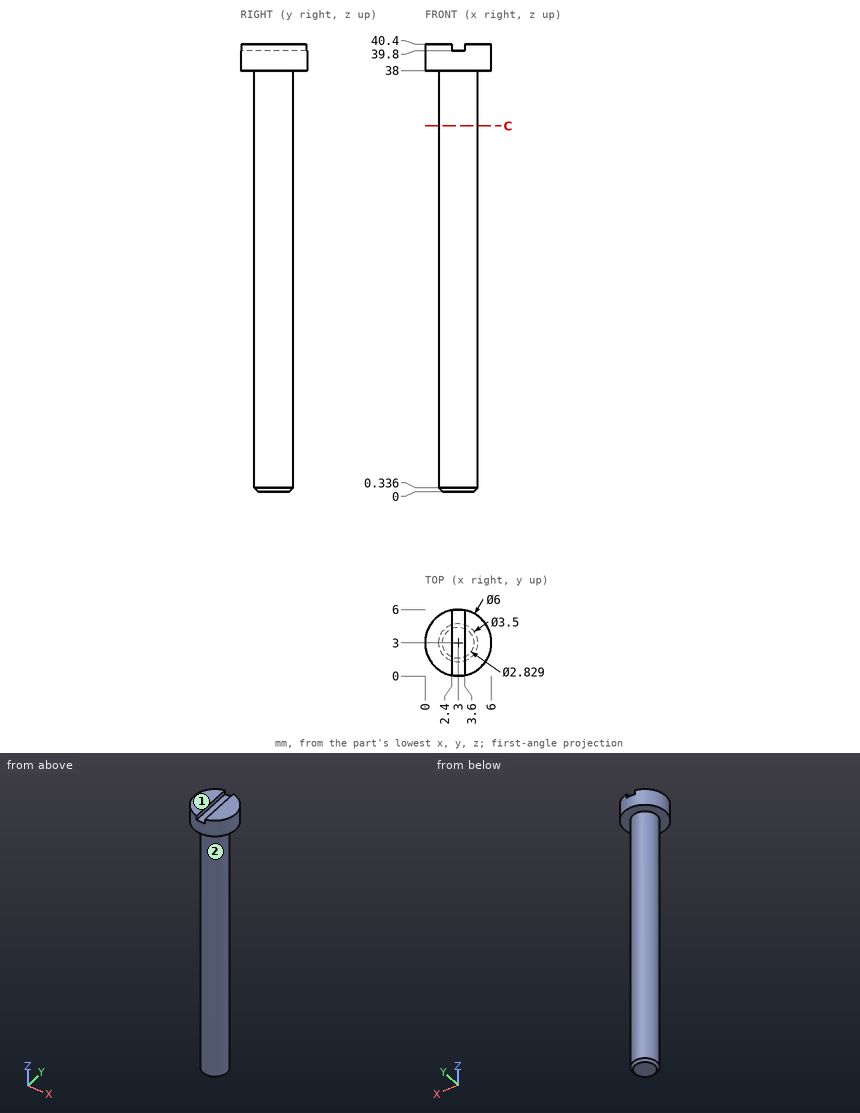
Geometry check sheet. Reference: drawing and pictorial views, mm from the part's lowest x, y, z. Round coordinates to 2 decimals unless told otherwise and drop trailing zeros. Order: outer loops, then holes, each group sorted by start corner. A loop starts at its lowest first (then second) coordinate and runs counter-clockwise, first axis right, second up. Notation, with made-up numbers: M 37,40 L 68,40 A32 cw 68,74 Z; hole C -19.75,79.25 d9. An arc over 180 degrees is marked long. Answer in a Markdown table with one row per item.
(1) Draft check along Z on the marked faces 1 and 2. Enter one of: released by +Z, released by -Z, zero draft, split by the parting line, or undercut.
Responses:
| item | result |
|---|---|
| face 1 | released by +Z |
| face 2 | zero draft |
(2) Go/stop test with flat-tipped pins: P1, Ø0.5, axis at y = 3.5, z = 40, coming from the +X side; P2, Ø0.6, axis at x = 3, y = 3, coming from the +Z side; P3, Ø0.7, axis at y = 1.5, z = 40, coming from the -X side. Record where each tip stops, or that it passes through.
Responses:
| item | result |
|---|---|
| P1 | stops at x = 5.99 |
| P2 | stops at z = 39.8 |
| P3 | stops at x = 0.23 |
(3) Scan lines: probe 1 along Z at (x, y) = (1.1, 2.65); probe 2 along Z at (x, y) = (2.7, 1.1); probe 3 along Y at (x, z) = (2.75, 6.5). Record each from-to range of solid material in increasing order. Write a range as from..to.
Responses:
| item | result |
|---|---|
| probe 1 | z = 38..40.4 |
| probe 2 | z = 38..39.8 |
| probe 3 | y = 1.27..4.73 |
(4) Sectioned sample at C-C, the plane z = 33. Record the cut outline in (x, y).
Responses:
| item | result |
|---|---|
| outline | C 3,3 d3.5 |
